Build history of the part. All positions in model axes, mm. Face numbers are marked on the shaded views. Give positions to 0.01 mm unless a question says otherwise; leave off trailing zeros. Loops run counter-clockwise (first coordinate to the right, second up) from the corner with the lowest first, then second, coordinate; pieces in that order, holes last. Notation, with made-up numbers: (-4, -9.75) -> (10, -9.75) arc R21 cw to (10, 26.25) -> close; hole circle Ø5 at (69.5, -6). An arc over 180 degrees is marked (long way). Answer in a Markdown table with one row per item. Add a question column.
Autodesk Inventor part; units mm, degrees
ref_plane "YZ Plane" through (0, 0, 0) normal (1, 0, 0) x (0, 1, 0)
ref_plane "XZ Plane" through (0, 0, 0) normal (0, 1, 0) x (-1, 0, 0)
ref_plane "XY Plane" through (0, 0, 0) normal (0, 0, 1) x (1, 0, 0)
sketch "Sketch2" plane through (0, 0, 0) normal (0, 0, 1) x (1, 0, 0)
  circle A0 centre (0, 0) radius 19.05
  circle A1 centre (0, 0) radius 22.225
  dimension "d0" = 38.1
  dimension "d1" = 3.175
extrude "Extrusion1" add sketch "Sketch2" along normal mid plane 195.98
sketch "Sketch3" plane through (0, 0, 97.99) normal (0, 0, -1) x (-1, 0, 0)
  circle A0 centre (0, 0) radius 22.225
  circle A1 centre (0, 0) radius 24.6
  dimension "d4" = 49.2
  dimension "d7" = 2.375
extrude "Extrusion2" add sketch "Sketch3" along normal blind 3.175
chamfer "Chamfer2" distance 2.3749 angle 45 1 edges at (-22.225, 0, 94.815)
properties part number "TUBE,1.5IN,ARM" material "Aluminum 7075"
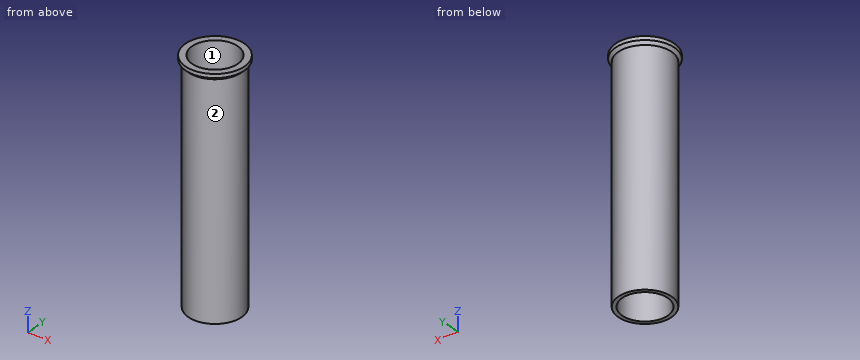
(1) Flat gauge pins, fed straight in: pin 1 Ø4 at (x, z) = (-17.5, 8.5) entering from -Y; pin 2 Ø3 at (y, z) = (-14.5, -2.5) entering from +X; pin 3 Ø5 at (x, z) = (5.5, -32) entering from +Y. Where does each tip first touch, or does it go through?
(2) Saw through at C-C, the plane z = 42. List the corners of the cut face in (x, y) (3 decimals).
(3) Wall check: line 1 along Y through (x, z) = (0, 43) (3 decimals); line 2 along X through (y, z) = (11.5, -37.5); line 3 along X through (y, z) = (-8.5, -74.5). Give the ranges that are in metal, low to high. Write a range as from..to.
(4) Two-plate mould, pull along Y, no slides. Class the marked faces 1 and 2: released by +Y, released by -Y, zero draft, split by the parting line, or undercut.
Worked answers:
| question | item | result |
|---|---|---|
| 1 | pin 1 | y = -15.93 |
| 1 | pin 2 | x = 18.03 |
| 1 | pin 3 | y = 22.02 |
| 2 | outline | circle Ø44.45 at (0, 0); hole circle Ø38.1 at (0, 0) |
| 3 | line 1 | -22.225..-19.05, 19.05..22.225 |
| 3 | line 2 | -19.02..-15.19, 15.19..19.02 |
| 3 | line 3 | -20.54..-17.05, 17.05..20.54 |
| 4 | face 1 | undercut |
| 4 | face 2 | split by the parting line |
